Build history of the part. All positions in model axes, mm. Round coordinates to 2 decimals unless told otherwise and drop trailing zeros. Loops run counter-clockwise (first coordinate to the right, second up) from the corner with the lowest first, then second, coordinate; pieces in that order, holes last. Notation, with made-up numbers: (56, -4) -> (71, -4) arc R13 ccw to (71, 12) -> close; hole circle Ø7 at (59.25, -15). An arc over 180 degrees is marked (long way). Put each result on its own line as item: value. Start each with the question number.
Item 1: Flat gauge pins, fed straight in: pin 1 Ø1.5 at (x, y) = (20.5, 39) entering from +Z; pin 2 Ø6 at (y, z) = (21.5, -26.5) entering from -X; pin 3 Ø3 at (y, z) = (18, -27) entering from +X. Where does each tip first touch, or does it go through?
Item 2: Drill centre lines: probe 1 along X at (y, z) = (13.5, -28); probe 2 along X at (y, z) = (14, -28.5); probe 3 along Z at (x, y) = (44, 47). Where is each one in solid material? Low to high. Write a range as [from, to].
Item 3: Pull direction X, two halves, no side cores. Call faces 1 (the cylindrical face through (22.1, 26.42, -30.48)), 2 (the flat face through (73.406, 26, -15)), 3 (the flat face through (36, 53.594, -15)), 4 (the cylindrical face through (58.69, 26.42, -3.04)): +X half, -X half, draft (parallel to the pull), parting line (faces both ways), or undercut.
Item 4: Cut at B-B, the plane x = 49.5. List the corners of the cut face in (y, z).
Item 5: Cut at C-C, the plane z = -26. List the corners of the cut face in (x, y), plus the area to 3 significant figures.
```python
from build123d import *

# Parameters (mm, degrees)
BOSS_EXTRUDE1_DEPTH = 53.594


with BuildPart() as part:
    # Sketch1 → Boss-Extrude1 (new body)
    with BuildSketch(Plane(origin=(0, 0, 0), x_dir=(1, 0, 0), z_dir=(0, 1, 0))):
        with BuildLine():
            Line((0, 23.139), (0, 7.341))
            ThreePointArc((0, 7.341), (4.531605435, 0.55884819), (12.531694095, 2.14995234))
            ThreePointArc((12.531694095, 2.14995234), (14.6815, 3.040388214), (16.831305905, 2.14995234))
            ThreePointArc((16.831305905, 2.14995234), (22.022, 0), (27.212694095, 2.14995234))
            ThreePointArc((27.212694095, 2.14995234), (29.3625, 3.040388214), (31.512305905, 2.14995234))
            ThreePointArc((31.512305905, 2.14995234), (36.703, 0), (41.893694095, 2.14995234))
            ThreePointArc((41.893694095, 2.14995234), (44.0435, 3.040388214), (46.193305905, 2.14995234))
            ThreePointArc((46.193305905, 2.14995234), (51.384, 0), (56.574694095, 2.14995234))
            ThreePointArc((56.574694095, 2.14995234), (58.7245, 3.040388214), (60.874305905, 2.14995234))
            ThreePointArc((60.874305905, 2.14995234), (68.874394565, 0.55884819), (73.406, 7.341))
            Line((73.406, 7.341), (73.406, 23.139))
            ThreePointArc((73.406, 23.139), (68.874394565, 29.92115181), (60.874305905, 28.33004766))
            ThreePointArc((60.874305905, 28.33004766), (58.7245, 27.439611786), (56.574694095, 28.33004766))
            ThreePointArc((56.574694095, 28.33004766), (51.384, 30.48), (46.193305905, 28.33004766))
            ThreePointArc((46.193305905, 28.33004766), (44.0435, 27.439611786), (41.893694095, 28.33004766))
            ThreePointArc((41.893694095, 28.33004766), (36.703, 30.48), (31.512305905, 28.33004766))
            ThreePointArc((31.512305905, 28.33004766), (29.3625, 27.439611786), (27.212694095, 28.33004766))
            ThreePointArc((27.212694095, 28.33004766), (22.022, 30.48), (16.831305905, 28.33004766))
            ThreePointArc((16.831305905, 28.33004766), (14.6815, 27.439611786), (12.531694095, 28.33004766))
            ThreePointArc((12.531694095, 28.33004766), (4.531605435, 29.92115181), (0, 23.139))
        make_face()
        with BuildLine():
            ThreePointArc((14.6815, 23.053321823), (14.682, 23.139), (14.6815, 23.224678177))
            ThreePointArc((14.6815, 23.224678177), (14.681, 23.139), (14.6815, 23.053321823))
        make_face(mode=Mode.SUBTRACT)
        with BuildLine():
            ThreePointArc((29.3625, 23.053321823), (29.363, 23.139), (29.3625, 23.224678177))
            ThreePointArc((29.3625, 23.224678177), (29.362, 23.139), (29.3625, 23.053321823))
        make_face(mode=Mode.SUBTRACT)
        with BuildLine():
            ThreePointArc((14.6815, 7.426678177), (14.681, 7.341), (14.6815, 7.255321823))
            ThreePointArc((14.6815, 7.255321823), (14.682, 7.341), (14.6815, 7.426678177))
        make_face(mode=Mode.SUBTRACT)
        with BuildLine():
            ThreePointArc((44.0435, 23.053321823), (44.044, 23.139), (44.0435, 23.224678177))
            ThreePointArc((44.0435, 23.224678177), (44.043, 23.139), (44.0435, 23.053321823))
        make_face(mode=Mode.SUBTRACT)
        with BuildLine():
            ThreePointArc((29.3625, 7.426678177), (29.362, 7.341), (29.3625, 7.255321823))
            ThreePointArc((29.3625, 7.255321823), (29.363, 7.341), (29.3625, 7.426678177))
        make_face(mode=Mode.SUBTRACT)
        with BuildLine():
            ThreePointArc((58.7245, 23.053321823), (58.725, 23.139), (58.7245, 23.224678177))
            ThreePointArc((58.7245, 23.224678177), (58.724, 23.139), (58.7245, 23.053321823))
        make_face(mode=Mode.SUBTRACT)
        with BuildLine():
            ThreePointArc((44.0435, 7.426678177), (44.043, 7.341), (44.0435, 7.255321823))
            ThreePointArc((44.0435, 7.255321823), (44.044, 7.341), (44.0435, 7.426678177))
        make_face(mode=Mode.SUBTRACT)
        with BuildLine():
            ThreePointArc((58.7245, 7.426678177), (58.724, 7.341), (58.7245, 7.255321823))
            ThreePointArc((58.7245, 7.255321823), (58.725, 7.341), (58.7245, 7.426678177))
        make_face(mode=Mode.SUBTRACT)
    extrude(amount=BOSS_EXTRUDE1_DEPTH)


solid = part.part
```
Reply:
1. pin 1: stops at z = -0.04
1. pin 2: stops at x = 0.01
1. pin 3: stops at x = 73.02
2. probe 1: x = [1.84, 12.92], [16.44, 27.6], [31.12, 42.28], [45.8, 56.97], [60.48, 71.57]
2. probe 2: x = [2.33, 12.36], [17.01, 27.04], [31.69, 41.72], [46.37, 56.4], [61.05, 71.08]
2. probe 3: z = [-27.44, -3.04]
3. face 1: undercut
3. face 2: +X half
3. face 3: draft
3. face 4: undercut
4. outline: (0, -30.23) -> (53.59, -30.23) -> (53.59, -0.25) -> (0, -0.25) -> close
5. outline: (0.58, 0) -> (72.83, 0) -> (72.83, 53.59) -> (0.58, 53.59) -> close
5. area: 3,870 mm^2
